Verification items for the finished model (mm, model axes). A direction names the side the tool comes from. Give positions to 0.01 mm unless a question says otherwise; leave off trailing zeros. Write each loop counter-clockwise with the first axis right and the second up, starting at its lowest first coordinate (ties: lowest second). Pieces come first, ordered by that corner, then holes.
from build123d import *

# Parameters (mm, degrees)
SKETCH1_R           = 11
BOSS_EXTRUDE1_DEPTH = 6.7
SKETCH2_R           = 3.9625
BOSS_EXTRUDE2_DEPTH = 2.7
SKETCH3_R           = 3.015
CUT_EXTRUDE1_DEPTH  = 19.175808098
SKETCH4_R           = 1.35
CUT_EXTRUDE2_DEPTH  = 17.937827488
SKETCH6_R           = 2
CUT_EXTRUDE3_DEPTH  = 17.937827488
CHAMFER1_SIZE       = 0.2
FILLET1_R           = 0.25


with BuildPart() as part:
    # Sketch1 → Boss-Extrude1 (new body)
    with BuildSketch(Plane.XY):
        Circle(SKETCH1_R)
    extrude(amount=-BOSS_EXTRUDE1_DEPTH)

    # Sketch2 → Boss-Extrude2 (add)
    with BuildSketch(Plane.XY):
        with Locations(Location((0, 0, 0), (0, 0, 180))):
            Circle(SKETCH2_R)
    extrude(amount=BOSS_EXTRUDE2_DEPTH)

    # Sketch3 → Cut-Extrude1 (cut, through all)
    with BuildSketch(Plane.XY.offset(2.7)):
        Circle(SKETCH3_R)
    extrude(amount=-CUT_EXTRUDE1_DEPTH, mode=Mode.SUBTRACT)

    # Sketch4 → Cut-Extrude2 (cut, through all)
    with BuildSketch(Plane.XY):
        with Locations((0, 8)):
            Circle(SKETCH4_R)
        with Locations((8, 0)):
            Circle(SKETCH4_R)
        with Locations((0, -8)):
            Circle(SKETCH4_R)
        with Locations((-8, 0)):
            Circle(SKETCH4_R)
    extrude(amount=-CUT_EXTRUDE2_DEPTH, mode=Mode.SUBTRACT)

    # Sketch6 → Cut-Extrude3 (cut, through all)
    with BuildSketch(Plane(origin=(0, 0, 0), x_dir=(0, 0, 1), z_dir=(-0.7071067811865487, -0.7071067811865465, 0))):
        with Locations(Location((-3.5, 0, 0), (0, 0, 270))):
            Circle(SKETCH6_R)
    extrude(amount=-CUT_EXTRUDE3_DEPTH, mode=Mode.SUBTRACT)

    # Chamfer1
    chamfer1_edges = [part.edges().sort_by_distance(p)[0] for p in [
        (-3.015, 0, -6.7),
        (-3.015, 0, 2.7),
    ]]
    chamfer(chamfer1_edges, length=CHAMFER1_SIZE)

    # Fillet1
    fillet1_edges = [part.edges().sort_by_distance(p)[0] for p in [
        (-11, 0, 0),
        (-11, 0, -6.7),
        (3.9625, 0, 2.7),
    ]]
    fillet(fillet1_edges, radius=FILLET1_R)


solid = part.part
Item 1: Sectioned sample at A-A on z = 1. Record the cut outline in (x, y) (1 decimal).
Answer key:
outline: circle Ø7.9 at (0, 0); hole circle Ø6 at (0, 0)
Item 2: Set-up check for faces 4 (the face through (-0.176, 9.339, -3.303)), 5 (the face through (0.52, -3.93, 1.21)): record each of +Z, -Z, +X, -X, +Y, -Y from which the full face is reachable in a straight line by a thin tool's end or side.
Answer key:
face 4: +Z, -Z
face 5: +Z
Item 3: Sectioned sample at C-C on y = 1. State how many separate pieces and enclosed holes the cut face has, then the cut area to 3 significant figures.
Answer key:
separate pieces: 4
enclosed holes: 0
area: 87.5 mm2
Item 4: Depth check by flat-ended pin: pin 1 (2 mm diameter, centred on x = 8, y = 0, fed in from -Z); pin 2 (5 mm diameter, centred on x = -3.5, z = -4.5, fed in from +Y); pin 3 (4 mm diameter, centred on y = -5.5, z = -2, fed in from +X); pin 4 (3.5 mm diameter, centred on x = 0, y = 8, fed in from +Z). Enter the tip coordinate at first touch or a pass-through.
Answer key:
pin 1: passes through
pin 2: stops at y = 10.95
pin 3: stops at x = 10.43
pin 4: stops at z = 0
Item 5: Scan lines: line 1 along Y through (x, z) = (0, -1.75) (3 decimals); line 2 along Z through (x, y) = (6, -2.25); line 3 along Z through (x, y) = (6, 8.25). Record each from-to range of solid material in increasing order.
Answer key:
line 1: y = -11 to -9.35, -6.65 to -3.015, 3.015 to 6.65, 9.35 to 11
line 2: z = -6.7 to 0
line 3: z = -6.7 to -4.71, -2.29 to 0
Item 6: Release check for a two-part mould opening along Z. For faces 1 (the face through (3.232, 6.058, -3.412)), 2 (the face through (9.288, 0.406, -3.303)), 3 (the face through (5, 0, 0)) record: released by +Z, released by -Z, zero draft, split by the parting line, or undercut.
Answer key:
face 1: undercut
face 2: zero draft
face 3: released by +Z
Item 7: Sectioned sample at B-B on z = -2.5. Record the cut outline in (x, y) (3 decimals), then the cut area to 3 significant figures.
Answer key:
outline: (0.52, 2.97) - (6.456, 8.906) arc R11 ccw (long way) to (8.906, 6.456) - (2.97, 0.52) arc R3.015 cw (long way) to start; hole circle Ø2.7 at (-8, 0); hole circle Ø2.7 at (0, -8); hole circle Ø2.7 at (0, 8); hole circle Ø2.7 at (8, 0)
area: 301 mm2
